Can you work these out from the model? Positions are in its coordinate system, mm. A direction names the side the tool comes from. Round coordinates to 2 decimals unless told otherwise and drop trailing zeros. Loops run counter-clockwise (first coordinate to the right, second up) from the corner with the lowest first, then second, coordinate; pieces in that order, holes last.
(1) I want a section at C-C on x = 0. Write out the boundary of the cut face in (y, z), plus the area to 3 significant figures.
(2) I want a section at D-D on x = 70.5. Write out the boundary of the cut face in (y, z).
(3) If I drill on line 1 along X through (y, z) = (-6, 0.8); line 2 along X through (y, z) = (-0.5, 0.1); line 3 along Y through (x, z) = (0, 0.8), over which ranges is the centre line in solid material (lowest first)?
(4) I want a section at A-A on y = 0. Write out the boundary of the cut face in (x, z), plus the area to 3 significant figures.
(5) Thinking about a two-plate mould opening in X: for faces 1 (the face through (26, 0, 2.5)), 2 (the face through (16.976, -4, 1)), 3 (the face through (79.541, -8, 1)), which applies, released by +X, released by -X, zero draft, split by the parting line, or undercut?
(6) Which directions (+Z, -Z, +X, -X, +Y, -Y) give clear straight access to the entire face, cutting with the end or side of a thin tool? Please do faces 4 (the face through (59, 4.5, 1)), 5 (the face through (27, 20.041, 1)), 6 (the face through (51, -5.5, 1)), 7 (the face through (73, -20.501, 1)), 8 (the face through (13.999, 12, 1)).
(7) Will these pins go through, and if not, where does the flat tip stop? pin 1 Ø0.8 at (x, z) = (-5.5, 1) entering from -Y; pin 2 Ø1.2 at (x, z) = (29.5, 1.5) entering from -Y; pin 3 Ø2 at (x, y) = (4.5, 6) entering from +Z; pin 4 Ø0.8 at (y, z) = (14.5, 0.5) entering from +X.
(8) I want a section at B-B on z = 2.1. Write out the boundary of the cut face in (x, y).
from build123d import *

# Parameters (mm, degrees)
F0_W      = 61.9999956
F0_H      = 10
F0_R      = 2.5
F1_DEPTH  = 2.5
F2_W      = 19.05
F2_H      = 4
F3_DEPTH  = 25.4
F4_R      = 1.27
F5_W      = 25
F5_H      = 2.5
F6_DEPTH  = 15.5406199982
F7_DEPTH  = 22.0406214
F8_W      = 12.99972
F8_H      = 2.5
F9_DEPTH  = 35.0012
F11_DEPTH = 22.0406214
F12_W     = 12.99972
F12_H     = 2.5
F13_DEPTH = 35.0012
F15_W     = 106.0812384
F15_H     = 37.9534307867
F16_DEPTH = 2.501


with BuildPart() as f1:
    # F0 (on Top) → F1 (new body)
    with BuildSketch(Plane.XY):
        with Locations((26.4999978, -0.5)):
            Rectangle(F0_W, F0_H)
        Circle(F0_R, mode=Mode.SUBTRACT)
        with Locations((52.9999956, 0)):
            Circle(F0_R, mode=Mode.SUBTRACT)
    extrude(amount=F1_DEPTH)

    # F2 (on face) → F3 (cut)
    with BuildSketch(Plane.XY.offset(2.5)):
        with Locations((26.5005656, -3.5)):
            Rectangle(F2_W, F2_H)
    extrude(amount=-F3_DEPTH, mode=Mode.SUBTRACT)

    # F4
    f4_edges = [f1.edges().sort_by_distance(p)[0] for p in [
        (36.025566, -1.5, 1.25),
        (16.975566, -1.5, 1.25),
    ]]
    fillet(f4_edges, radius=F4_R)

    # F5 (on face) → F6 (join)
    with BuildSketch(Plane(origin=(0, 4.5, 0), x_dir=(-1, 0, 0), z_dir=(0, 1, 0))):
        with Locations((-26.49943, 1.25)):
            Rectangle(F5_W, F5_H)
    extrude(amount=F6_DEPTH)

    # F7 (add): a face of the model
    f7_faces = [f1.faces().sort_by_distance(p)[0] for p in [
        (57.4999956, -0.5, 1.25),
    ]]
    extrude(f7_faces, amount=F7_DEPTH)

    # F8 (on face) → F9 (join)
    with BuildSketch(Plane.XZ.offset(5.5)):
        with Locations((73.040757, 1.25)):
            Rectangle(F8_W, F8_H)
    extrude(amount=F9_DEPTH)

    # F11 (add): a face of the model
    f11_faces = [f1.faces().sort_by_distance(p)[0] for p in [
        (-4.5, -0.5, 1.25),
    ]]
    extrude(f11_faces, amount=F11_DEPTH)

    # F12 (on face) → F13 (join)
    with BuildSketch(Plane.XZ.offset(5.5)):
        with Locations((-20.0407614, 1.25)):
            Rectangle(F12_W, F12_H)
    extrude(amount=F13_DEPTH)

    # F15 (on face) → F16 (cut, through all)
    with BuildSketch(Plane.XY.offset(2.5)):
        with Locations((26.4999978, -39.4779353934)):
            Rectangle(F15_W, F15_H)
    extrude(amount=-F16_DEPTH, mode=Mode.SUBTRACT)


solid = f1.part
Filled sheet:
1. outline: (-5.5, 0) - (-2.5, 0) - (-2.5, 2.5) - (-5.5, 2.5) - close; (2.5, 0) - (4.5, 0) - (4.5, 2.5) - (2.5, 2.5) - close
1. area: 12.5 mm2
2. outline: (-20.5, 0) - (4.5, 0) - (4.5, 2.5) - (-20.5, 2.5) - close
3. line 1: x = -26.54 to -13.54, 66.54 to 79.54
3. line 2: x = -26.54 to -2.45, 2.45 to 50.55, 55.45 to 79.54
3. line 3: y = -5.5 to -2.5, 2.5 to 4.5
4. outline: (-26.54, 0) - (-2.5, 0) - (-2.5, 2.5) - (-26.54, 2.5) - close; (2.5, 0) - (50.5, 0) - (50.5, 2.5) - (2.5, 2.5) - close; (55.5, 0) - (79.54, 0) - (79.54, 2.5) - (55.5, 2.5) - close
4. area: 240 mm2
5. face 1: zero draft
5. face 2: undercut
5. face 3: released by +X
6. face 4: +Z, -Z, +X, +Y
6. face 5: +Z, -Z, +X, -X, +Y
6. face 6: +Z, -Z, -Y
6. face 7: +Z, -Z, +X, -X, -Y
6. face 8: +Z, -Z, -X, +Y
7. pin 1: stops at y = -5.5
7. pin 2: stops at y = -1.5
7. pin 3: passes through
7. pin 4: stops at x = 39
8. outline: (-26.54, -20.5) - (-13.54, -20.5) - (-13.54, -5.5) - (16.98, -5.5) - (16.98, -2.77) arc R1.27 cw to (18.25, -1.5) - (34.76, -1.5) arc R1.27 cw to (36.03, -2.77) - (36.03, -5.5) - (66.54, -5.5) - (66.54, -20.5) - (79.54, -20.5) - (79.54, 4.5) - (39, 4.5) - (39, 20.04) - (14, 20.04) - (14, 4.5) - (-26.54, 4.5) - close; hole circle Ø5 at (0, 0); hole circle Ø5 at (53, 0)
